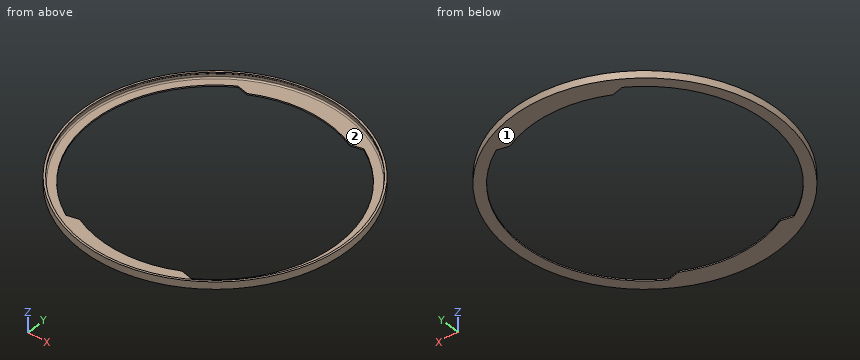
Autodesk Fusion 360 part; units mm, degrees
sketch "Ring" plane through (0, 0, 0) normal (1, 0, 0) x (0, 1, 0)
  line L0 (0, 0) -> (0, 5.5)
  line L1 (0, 0) -> (14, 0)
  line L2 (14, 0) -> (14, 1)
  line L3 (14, 1) -> (1, 1)
  line L4 (1, 1) -> (1, 4)
  line L5 (1, 4) -> (1.5, 4.5)
  line L6 (1.5, 4.5) -> (1.5, 5.5)
  line L7 (0, 5.5) -> (1.5, 5.5)
  line L8 (101, -11) -> (101, 21) construction
  point P0 (101, 0)
  dimension "d11" = 1
  dimension "d12" = 3
  dimension "d13" = 1
  dimension "d21" = 1
  dimension "d44" = 135
  dimension "d45" = 0.5
  dimension "d47" = 13
  dimension "d48" = 100
revolve "Revolve Ring" add sketch "Ring" angle 360 about axis through (0, 101, -11) along (0, 0, 1)
sketch "Cutout" plane through (0, 0, 1) normal (0, 0, 1) x (-1, 0, 0)
  circle A0 centre (0, -101) radius 100
  circle A1 centre (0, -101) radius 87
  circle A2 centre (0, -101) radius 87
  circle A3 centre (0, -101) radius 93
  line L0 (39.1124, -23.2876) -> (47.8845, -21.275)
  line L1 (-38.6062, -23.0349) -> (-47.365, -20.9653)
  line L2 (-38.6062, -178.9651) -> (-47.365, -181.0347)
  line L3 (39.1124, -178.7124) -> (47.8845, -180.725)
  line L4 (47.8845, -180.725) -> (47.8845, -21.275) construction
  line L5 (-47.365, -181.0347) -> (-47.365, -20.9653) construction
  point P0 (39.1124, -23.2876)
  dimension "d24" = 0
  dimension "d25" = 186
  dimension "d37" = 9
  dimension "d49" = 95.25
  dimension "d50" = 77.719
  dimension "d52" = 159.45
extrude "Remove Cutout" cut sketch "Cutout" against normal blind 10 contours A1 A2 A3 L0 L3 | A1 A2 A3 L1 L2
fillet "Fillet2" radius 1 1 edges at (-93.2327, 64.8385, 1)
equation "d11 = bottom_thickness"
equation "d12 = cardboard_thickness"
equation "d21 = edge_thickness"
equation "d25 = spool_diameter - ( 2 * width_to_holes )"
equation "bottom_thickness = 1 mm"
equation "cardboard_thickness = 3 mm"
equation "spool_diameter = 200 mm"
equation "edge_thickness = 1 mm"
equation "width_to_holes = 7 mm"
equation "total_width = 13 mm"
equation "d47 = total_width"
equation "d48 = spool_diameter / 2"
equation "fillet_radius = 1 mm"
The listing builds one solid part. Answer for the finished solid, in the listing's coordinates (mm). Face numbers are marked on the shaded views. Coordinates: 2 decimals unless noted, no trailing zeros. Loops run counter-clockwise (first coordinate to the right, second up) from the corner with the lowest first, then second, coordinate; pieces in that order, holes last. Notation, with made-up numbers: (85.25, 72) - (113.25, 72) arc R6 cw to (113.25, 79) - close; hole circle Ø6 at (56, -16). An arc over 180 degrees is marked (long way). Use a Markdown table: item, result. Add a question column.
1) The mould has two halves that part along Y. Classify the marked faces 1 and 2: released by +Y, released by -Y, zero draft, split by the parting line, or undercut.
2) Given pin 1 (1 mm diameter, centred on x = -39.5, z = 3, fed in from -Y); pin 2 (3 mm diameter, centred on y = 172, z = 3, fed in from +X); pin 3 (1.5 mm diameter, centred on x = -57.5, z = 2, fed in from -Y), each flat-ended and moving along its own axis, determine where each tip first touches the part or whether it passes through.
3) The part is cut by section A-A, the plane y = 101. Give the vertices of the cut face in (x, z).
4) The part is cut by section B-B, the plane x = 0. Give the vertices of the cut face in (y, z).
5) Find the intervals of material crossed by line 1 (X direction, y = 101, z = 5.15); line 2 (X direction, y = 101, z = 2.6); line 3 (Z direction, x = 93, y = 93), in increasing order.
6) The part is cut by section C-C, the plane z = 2.95. Give the vertices of the cut face in (x, y).
Here are the results:
| question | item | result |
|---|---|---|
| 1 | face 1 | zero draft |
| 1 | face 2 | undercut |
| 2 | pin 1 | stops at y = 7.83 |
| 2 | pin 2 | stops at x = 73.29 |
| 2 | pin 3 | stops at y = 17.45 |
| 3 | outline | (-101, 0) - (-93, 0) - (-93, 1) - (-99, 1) arc R1 cw to (-100, 2) - (-100, 4) - (-99.5, 4.5) - (-99.5, 5.5) - (-101, 5.5) - close; (93, 0) - (101, 0) - (101, 5.5) - (99.5, 5.5) - (99.5, 4.5) - (100, 4) - (100, 2) arc R1 cw to (99, 1) - (93, 1) - close |
| 4 | outline | (0, 0) - (14, 0) - (14, 1) - (2, 1) arc R1 cw to (1, 2) - (1, 4) - (1.5, 4.5) - (1.5, 5.5) - (0, 5.5) - close; (188, 0) - (202, 0) - (202, 5.5) - (200.5, 5.5) - (200.5, 4.5) - (201, 4) - (201, 2) arc R1 cw to (200, 1) - (188, 1) - close |
| 5 | line 1 | x = -101 to -99.5, 99.5 to 101 |
| 5 | line 2 | x = -101 to -100, 100 to 101 |
| 5 | line 3 | z = 0 to 1 |
| 6 | outline | circle Ø202 at (0, 101); hole circle Ø200 at (0, 101) |
